Part model, mm, in its own coordinate system. Face numbers are marked on the shaded views. A direction names the side the tool comes from. Give positions to 0.01 mm unless a question says otherwise; leave off trailing zeros. Write each loop counter-clockwise with the first axis right and the second up, starting at its lowest first coordinate (ties: lowest second). Pieces come first, ordered by that corner, then holes. Notation, with made-up numbers: M -32,-10 L -7,-10 A31 cw -7,20 Z; hole C -10,28.25 d9. An arc over 180 degrees is marked long. Use a Markdown table: item, result.
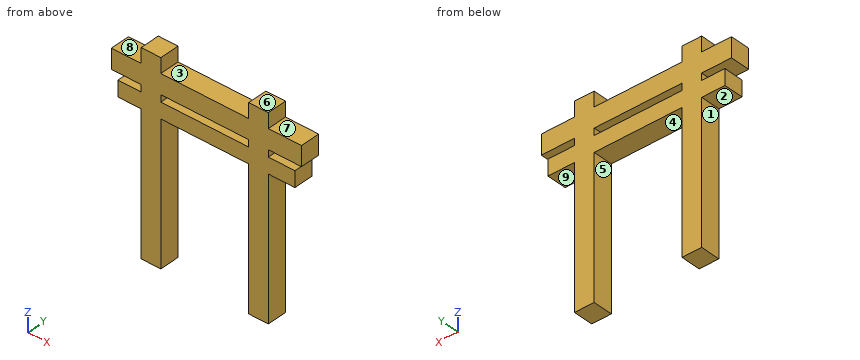
```python
from build123d import *

# Parameters (mm, degrees)
F0_W     = 15
F0_H     = 15
F1_DEPTH = 150
F3_W     = 135
F3_H     = 12
F4_DEPTH = 7.5
F5_W     = 145
F5_H     = 15
F6_DEPTH = 7.5


with BuildPart() as f1:
    # F0 (on Top) → F1 (new body)
    with BuildSketch(Plane.XY):
        with Locations((-42.26087, 0)):
            Rectangle(F0_W, F0_H)
        with Locations((39.717395, 0)):
            Rectangle(F0_W, F0_H)
    extrude(amount=F1_DEPTH)


with BuildPart() as f1_1:
    # F2: moved
    add(f1.part.moved(Location((0, 0, -75.4))))

    # F3 (on Front) → F4 (join, symmetric)
    with BuildSketch(Plane.XZ):
        with Locations((0, 37.059784)):
            Rectangle(F3_W, F3_H)
    extrude(amount=F4_DEPTH, both=True)

    # F5 (on Front) → F6 (join, symmetric)
    with BuildSketch(Plane.XZ):
        with Locations((0, 55.807658)):
            Rectangle(F5_W, F5_H)
    extrude(amount=F6_DEPTH, both=True)


solid = f1_1.part
```
1. Cut at A-A, the plane x = -19.5. Give the cut face in (y, z), then the cut area to 3 significant figures.
Findings below:
| item | result |
|---|---|
| outline | M -7.5,31.06 L 7.5,31.06 L 7.5,43.06 L -7.5,43.06 Z; M -7.5,48.31 L 7.5,48.31 L 7.5,63.31 L -7.5,63.31 Z |
| area | 405 mm2 |
2. Cut at B-B, the plane z = -39. Give the cut face in (x, y).
Findings below:
| item | result |
|---|---|
| outline | M -49.76,-7.5 L -34.76,-7.5 L -34.76,7.5 L -49.76,7.5 Z; M 32.22,-7.5 L 47.22,-7.5 L 47.22,7.5 L 32.22,7.5 Z |
3. Drill centre lines: L1, parallel to X at y = -7, z = 9; L2, parallel to Z at x = -3.5, y = 2.75. Where is each one in solid material? Low to high.
Findings below:
| item | result |
|---|---|
| L1 | -49.76 to -34.76, 32.22 to 47.22 |
| L2 | 31.06 to 43.06, 48.31 to 63.31 |
4. Drop flat-ended pins along their axis: P1, Ø4, axis at y = 0.5, z = -9, coming from the +X side; P2, Ø1, axis at y = -4, z = 37.5, coming from the -X side; P3, Ø2.5, axis at y = -2.5, z = 46.5, coming from the -X side. Give the stop position or say it passes through.
Findings below:
| item | result |
|---|---|
| P1 | x = 47.22 |
| P2 | x = -67.5 |
| P3 | x = -49.76 |
5. Tool access for the marked faces 5, 6, 7, 8 and 9: list every direction of +Z, -Z, +X, -X, +Y, -Y with a clear straight run to the whole face (end or side of a thin tool).
Findings below:
| item | result |
|---|---|
| face 5 | -Z, +Y, -Y |
| face 6 | +Z, +X, -X, +Y, -Y |
| face 7 | +Z, +X, +Y, -Y |
| face 8 | +Z, -X, +Y, -Y |
| face 9 | -Z, +X, +Y, -Y |
6. Two-plate mould, pull along X, no slides. Class the marked faces 1, 2, 3 and 4: released by +X, released by -X, zero draft, split by the parting line, or undercut.
Findings below:
| item | result |
|---|---|
| face 1 | released by -X |
| face 2 | zero draft |
| face 3 | undercut |
| face 4 | undercut |
